Autodesk Inventor part; units mm, degrees
ref_plane "YZ Plane" through (0, 0, 0) normal (1, 0, 0) x (0, 1, 0)
ref_plane "XZ Plane" through (0, 0, 0) normal (0, 1, 0) x (-1, 0, 0)
ref_plane "XY Plane" through (0, 0, 0) normal (0, 0, 1) x (1, 0, 0)
sketch "Эскиз1" plane through (0, 0, 0) normal (0, 0, 1) x (1, 0, 0)
  line L0 (7.5, -5) -> (7.5, 0)
  line L1 (5.0577, -5) -> (7.5, -5)
  line L2 (5.0577, -5) -> (-4.3392, -5)
  line L3 (-6.7815, -5) -> (-4.3392, -5)
  line L4 (-6.7815, -5) -> (-6.7815, 0)
  line L5 (-6.7815, 0) -> (-4.3392, 0)
  line L6 (5.0577, 0) -> (-4.3392, 0)
  line L7 (5.0577, 0) -> (7.5, 0)
  line L8 (7.5, -10.5) -> (-7.5, -10.5)
  line L9 (7.5, 0) -> (-6.7815, 0)
  line L10 (7.5, 10.5) -> (7.5, 0)
  line L11 (-7.5, 10.5) -> (7.5, 10.5)
  line L12 (-7.5, -10.5) -> (-7.5, 10.5)
  line L13 (7.5, -10.5) -> (-7.5, -10.5)
  line L14 (7.5, -5) -> (7.5, -10.5)
  line L15 (7.5, -5) -> (-6.7815, -5)
  line L16 (-6.7815, -5) -> (-6.7815, 0)
  point P0 (0, 0)
extrude "Выдавливание1" add sketch "Эскиз1" along normal blind 10 contours L14 L8 L12 L11 L10 L7 L6 L5 L4 L3 L2 L1
sketch "Эскиз2" plane through (-7.5, 10.5, 0) normal (0, 1, 0) x (1, 0, 0)
  circle A0 centre (7.8593, -5) radius 2
  point P0 (7.5, 0)
extrude "Выдавливание2" cut sketch "Эскиз2" against normal through all
sketch "Эскиз3" plane through (-7.5, 10.5, 0) normal (0, 1, 0) x (1, 0, 0)
  line L0 (15, -10) -> (0, -10)
  line L1 (15, -10) -> (15, -16.9946)
  line L2 (15, -16.9946) -> (0, -10)
  point P0 (7.5, 0)
  dimension "d5" = 25
extrude "Выдавливание3" add sketch "Эскиз3" against normal up to surface (21 mm away)
sketch "Эскиз4" plane through (7.5, -10.5, 16.9946) normal (-0.4226183, 0, 0.9063078) x (0.9063078, 0, 0.4226183)
  line L0 (-16.5507, 0) -> (0, 0)
  line L1 (0, 21) -> (0, 0)
  line L2 (-16.5507, 21) -> (0, 21)
  line L3 (-16.5507, 21) -> (-16.5507, 0)
  line L4 (-18.2753, -1.7247) -> (1.7247, -1.7247)
  line L5 (1.7247, -1.7247) -> (1.7247, 22.7247)
  line L6 (1.7247, 22.7247) -> (-18.2753, 22.7247)
  line L7 (-18.2753, 22.7247) -> (-18.2753, -1.7247)
  point P0 (-13.9795, 10.5)
  dimension "d8" = 20
extrude "Выдавливание4" add sketch "Эскиз4" along normal blind 2 contours L3 L2 L1 L0 | L7 L6 L5 L4
sketch "Эскиз5" plane through (6.6548, -10.5, 18.8072) normal (-0.4226183, 0, 0.9063078) x (0.9063078, 0, 0.4226183)
  line L0 (0.2247, 19) -> (-16.7753, 19)
  line L1 (-16.7753, 19) -> (-16.7753, 2)
  line L2 (-16.7753, 2) -> (0.2247, 2)
  line L3 (0.2247, 2) -> (0.2247, 19)
  line L4 (1.7247, -1.7247) -> (1.7247, 22.7247)
  line L5 (-18.2753, -1.7247) -> (1.7247, -1.7247)
  line L6 (-0.7753, 18) -> (-15.7753, 18)
  line L7 (-15.7753, 18) -> (-15.7753, 3)
  line L8 (-15.7753, 3) -> (-0.7753, 3)
  line L9 (-0.7753, 3) -> (-0.7753, 18)
  point P0 (-13.9795, 10.5)
  point P1 (0.2247, 10.5)
  point P2 (1.7247, 10.5)
  point P3 (-8.2753, 2)
  point P4 (-8.2753, -1.7247)
  dimension "d11" = 17
  dimension "d12" = 1
extrude "Выдавливание5" add sketch "Эскиз5" along normal blind 8
fillet "Сопряжение1" radius 2 8 edges at (5.1679, -8.5, 22.5274) (5.1679, 8.5, 22.5274) (-10.2393, 8.5, 15.3429) (-10.2393, -8.5, 15.3429) (-9.333, 7.5, 15.7655) (4.2616, 7.5, 22.1048) (-9.333, -7.5, 15.7655) (4.2616, -7.5, 22.1048)
sketch "Эскиз6" plane through (7.5, 0, 0) normal (1, 0, 0) x (0, 0, -1)
  point P0 (0, 0)
equation "\"degg\" = 65deg"
properties part number "base_65"
The listing builds one solid part. Answer for the finished solid, in the listing's coordinates (mm). A direction names the side the tool comes from. Round coordinates to 2 decimals unless told otherwise and drop trailing zeros. Write each loop counter-clockwise with the first axis right and the second up, starting at its lowest first coordinate (ties: lowest second). Pieces come first, ordered by that corner, then holes. Notation, with made-up numbers: (27, -22) -> (81, -22) arc R18 ccw to (81, 8) -> close; hole circle Ø7 at (18, 89.25). An arc over 180 degrees is marked (long way). Answer as a JSON object with one key per item and string values. Group by question number.
Q1. Section A-A (z = 5) is taken. Write down the section's boundary in (x, y), plus the area to 3 significant figures.
Q2. Straight lines are drawn through the part: line 1 along Y through (x, z) = (3.75, 7.5); line 2 along Y through (x, z) = (0.5, 20); line 3 along X through (y, z) = (3.25, 5). For each, find the intervals that lie inside material, in ascending order.
Q3. Which of the six approach directions +Z, -Z, +X, -X, +Y, -Y give full straight-line access (tool end or side, diameter ignored) to faces 5 (the face through (0, 10.5, 8)), 6 (the face through (-9.309, 0.077, 15.715)), 7 (the face through (4.6, -7.93, 22.32)), 8 (the face through (-2, 8.5, 19)), 9 (the face through (0, -10.5, 8))?
Q4. Determine the mould class of faces 1 (the face through (8.646, -0.171, 18.617)), 2 (the face through (3.72, 6.9, 21.91)), 3 (the face through (0.3, -5, 2.7)), 4 (the face through (-9.72, 7.93, 15.65)) for opening direction X: pulls with the +X half, pulls with the -X half, needs draft (parallel to the pull), parting line crosses it, or undercut.
Q5. Section B-B (x = -0.75) is taken. Write down the section's boundary in (y, z), plus the area to 3 significant figures.
Q6. Each of these flat-tipped pins is pushed along its axis until it touches: pin 1 Ø4 at (x, y) = (-2.5, -2.5) entering from -Z; pin 2 Ø4 at (y, z) = (3.5, 5.5) entering from -X; pin 3 Ø8 at (y, z) = (-8.5, 12.5) entering from -X. Where does it stop, or does it pass through?
Check values:
{
 "1": {"outline": "(-7.5, -10.5) -> (-1.64, -10.5) -> (-1.64, -5) -> (-6.78, -5) -> (-6.78, 0) -> (-1.64, 0) -> (-1.64, 10.5) -> (-7.5, 10.5) -> close; (2.36, -10.5) -> (7.5, -10.5) -> (7.5, -5) -> (2.36, -5) -> close; (2.36, 0) -> (7.5, 0) -> (7.5, 10.5) -> (2.36, 10.5) -> close", "area": "180 mm^2"},
 "2": {"line 1": "-10.5 to -5, 0 to 10.5", "line 2": "-8.5 to -7.5, 7.5 to 8.5", "line 3": "-7.5 to -1.64, 2.36 to 7.5"},
 "3": {"face 5": "-Z, +X, +Y", "face 6": "+Z", "face 7": "+Z, -Y", "face 8": "+Z, -X, +Y", "face 9": "-Z, +X, -Y"},
 "4": {"face 1": "pulls with the +X half", "face 2": "undercut", "face 3": "needs draft", "face 4": "pulls with the -X half"},
 "5": {"outline": "(-12.22, 13.15) -> (-10.5, 13.15) -> (-10.5, 6.66) -> (-5, 6.66) -> (-5, 10) -> (0, 10) -> (0, 6.66) -> (10.5, 6.66) -> (10.5, 13.15) -> (12.22, 13.15) -> (12.22, 15.35) -> (8.5, 15.35) -> (8.5, 24.18) -> (7.5, 24.18) -> (7.5, 15.35) -> (-7.5, 15.35) -> (-7.5, 24.18) -> (-8.5, 24.18) -> (-8.5, 15.35) -> (-12.22, 15.35) -> close; (-10.5, 0) -> (-5, 0) -> (-5, 3.34) -> (-10.5, 3.34) -> close; (0, 0) -> (10.5, 0) -> (10.5, 3.34) -> (0, 3.34) -> close", "area": "244 mm^2"},
 "6": {"pin 1": "z = 10", "pin 2": "x = -7.5", "pin 3": "x = -10.58"}
}
